Read the model definition and answer for the solid it produces. Units are mm, in the model's axes. A direction names the side the tool comes from. Coordinates: 2 decimals unless noted, no trailing zeros. Write each loop counter-clockwise with the first axis right and the second up, starting at its lowest first coordinate (ties: lowest second). Pieces come first, ordered by that corner, then holes.
(1) The part is cut by section C-C, the plane z = -15. Determine the outline of the cut face in (x, y), and give its area (3 significant figures).
(2) The part is cut by section B-B, the plane x = 15. Determine the outline of the cut face in (y, z), and give its area (3 significant figures).
(3) The part is cut by section D-D, the plane z = -6. Determine the outline of the cut face in (x, y).
(4) Given pin 1 (1.2 mm diameter, centred on y = 3, z = 9.5, fed in from +X); pin 2 (2 mm diameter, centred on y = 3.5, z = -4, fed in from -X); pin 3 (18.5 mm diameter, centred on x = -4, z = -3, fed in from +Y), each flat-ended and moving along its own axis, determine where each tip first touches the part or whether it passes through.
(5) The part is cut by section A-A, the plane y = 2.85. Determine the outline of the cut face in (x, z).
(6) Straight lines are drawn through the part: line 1 along X through (y, z) = (4.55, 15); line 2 along X through (y, z) = (0.75, 0); line 3 along X through (y, z) = (3.1, -15). For each, find the intervals that lie inside material, in ascending order.
(7) Which of the six approach directions +Z, -Z, +X, -X, +Y, -Y give full straight-line access (tool end or side, diameter ignored) to faces 4 (the flat face through (-20, 3, 0)), 5 (the cylindrical face through (-14.052, 3.472, 16.237)), 6 (the flat face through (0, 2, -19))?
(8) Determine the mould class of faces 1 (the flat face through (10, 4, -19)), 2 (the flat face through (26.9, 0.7, 10.8)), 3 (the cylindrical face through (14.052, 3.472, 13.763)) for opening direction Z: pulls with the +Z half, pulls with the -Z half, needs draft (parallel to the pull), parting line crosses it, or undercut.
```python
from build123d import *

# Parameters (mm, degrees)
SKETCH1_R           = 1.5
SKETCH1_R_2         = 2.5
BOSS_EXTRUDE1_DEPTH = 1.5
SKETCH2_W           = 40
SKETCH2_H           = 40
SKETCH2_R           = 1.5
SKETCH2_R_2         = 1.558204887
BOSS_EXTRUDE2_DEPTH = 4
SKETCH3_W           = 20
SKETCH3_H           = 3.5
CUT_EXTRUDE1_DEPTH  = 2
SKETCH4_W           = 20
SKETCH4_H           = 3.5
CUT_EXTRUDE2_DEPTH  = 2
FILLET1_R           = 3


with BuildPart() as part:
    # Sketch1 → Boss-Extrude1 (new body)
    with BuildSketch(Plane(origin=(0, 0, 0), x_dir=(1, 0, 0), z_dir=(0, 1, 0))):
        Polygon((-20, 20), (20, 20), (35, 0), (20, -20), (-20, -20), (-35, 0), align=None)
        with Locations(Location((-15, 15, 0), (0, 0, 270))):
            Circle(SKETCH1_R, mode=Mode.SUBTRACT)
        with Locations(Location((15, 15, 0), (0, 0, 270))):
            Circle(SKETCH1_R, mode=Mode.SUBTRACT)
        with Locations(Location((15, -15, 0), (0, 0, 90))):
            Circle(SKETCH1_R, mode=Mode.SUBTRACT)
        with Locations(Location((-15, -15, 0), (0, 0, 90))):
            Circle(SKETCH1_R, mode=Mode.SUBTRACT)
        with Locations(Location((-30, 0, 0), (0, 0, 270))):
            Circle(SKETCH1_R_2, mode=Mode.SUBTRACT)
        with Locations(Location((30, 0, 0), (0, 0, 90))):
            Circle(SKETCH1_R_2, mode=Mode.SUBTRACT)
    extrude(amount=BOSS_EXTRUDE1_DEPTH)

    # Sketch2 → Boss-Extrude2 (add)
    with BuildSketch(Plane(origin=(0, 1.5, 0), x_dir=(1, 0, 0), z_dir=(0, 1, 0))):
        Rectangle(SKETCH2_W, SKETCH2_H)
        with Locations(Location((-15, 15, 0), (0, 0, 270))):
            Circle(SKETCH2_R, mode=Mode.SUBTRACT)
        with Locations(Location((15, -15, 0), (0, 0, 270))):
            Circle(SKETCH2_R_2, mode=Mode.SUBTRACT)
        with Locations(Location((-15, -15, 0), (0, 0, 90))):
            Circle(SKETCH2_R_2, mode=Mode.SUBTRACT)
        with Locations(Location((15, 15, 0), (0, 0, 90))):
            Circle(SKETCH2_R, mode=Mode.SUBTRACT)
        with BuildLine():
            Line((-18.5, 11.429285786), (-18.5, -11.429285786))
            ThreePointArc((-18.5, -11.429285786), (-11.464466094, -11.464466094), (-11.429285786, -18.5))
            Line((-11.429285786, -18.5), (11.429285786, -18.5))
            ThreePointArc((11.429285786, -18.5), (11.464466094, -11.464466094), (18.5, -11.429285786))
            Line((18.5, -11.429285786), (18.5, 11.429285786))
            ThreePointArc((18.5, 11.429285786), (11.464466094, 11.464466094), (11.429285786, 18.5))
            Line((11.429285786, 18.5), (-11.429285786, 18.5))
            ThreePointArc((-11.429285786, 18.5), (-11.464466094, 11.464466094), (-18.5, 11.429285786))
        make_face(mode=Mode.SUBTRACT)
    extrude(amount=BOSS_EXTRUDE2_DEPTH)

    # Sketch3 → Cut-Extrude1 (cut)
    with BuildSketch(Plane.XY.offset(20)):
        with Locations((0, 3.75)):
            Rectangle(SKETCH3_W, SKETCH3_H)
    extrude(amount=-CUT_EXTRUDE1_DEPTH, mode=Mode.SUBTRACT)

    # Sketch4 → Cut-Extrude2 (cut)
    with BuildSketch(Plane(origin=(0, 0, -20), x_dir=(-1, 0, 0), z_dir=(0, 0, -1))):
        with Locations((0, 3.75)):
            Rectangle(SKETCH4_W, SKETCH4_H)
    extrude(amount=-CUT_EXTRUDE2_DEPTH, mode=Mode.SUBTRACT)

    # Fillet1
    fillet1_edges = [part.edges().sort_by_distance(p)[0] for p in [
        (-35, 0.75, 0),
        (35, 0.75, 0),
    ]]
    fillet(fillet1_edges, radius=FILLET1_R)


solid = part.part
```
Computed:
1. outline: (-23.75, 0) - (-16.5, 0) - (-16.5, 5.5) - (-20, 5.5) - (-20, 1.5) - (-23.75, 1.5) - close; (-13.5, 0) - (13.5, 0) - (13.5, 5.5) - (10, 5.5) - (10, 1.5) - (-10, 1.5) - (-10, 5.5) - (-13.5, 5.5) - close; (16.5, 0) - (23.75, 0) - (23.75, 1.5) - (20, 1.5) - (20, 5.5) - (16.5, 5.5) - close
1. area: 118 mm2
2. outline: (0, -20) - (5.5, -20) - (5.5, -16.5) - (0, -16.5) - close; (0, -13.5) - (5.5, -13.5) - (5.5, -10) - (1.5, -10) - (1.5, 10) - (5.5, 10) - (5.5, 13.44) - (1.5, 13.44) - (1.5, 13.5) - (0, 13.5) - close; (0, 16.5) - (1.5, 16.5) - (1.5, 16.56) - (5.5, 16.56) - (5.5, 20) - (0, 20) - close
2. area: 107 mm2
3. outline: (-30.5, 0) - (30.5, 0) - (30.5, 1.5) - (20, 1.5) - (20, 5.5) - (18.5, 5.5) - (18.5, 1.5) - (-18.5, 1.5) - (-18.5, 5.5) - (-20, 5.5) - (-20, 1.5) - (-30.5, 1.5) - close
4. pin 1: stops at x = 20
4. pin 2: stops at x = -20
4. pin 3: stops at y = 1.5
5. outline: (-20, -20) - (-10, -20) - (-10, -18.5) - (-11.43, -18.5) arc R5 ccw to (-18.5, -11.43) - (-18.5, 11.43) arc R5 ccw to (-11.43, 18.5) - (-10, 18.5) - (-10, 20) - (-20, 20) - close; (10, -20) - (20, -20) - (20, 20) - (10, 20) - (10, 18.5) - (11.43, 18.5) arc R5 ccw to (18.5, 11.43) - (18.5, -11.43) arc R5 ccw to (11.43, -18.5) - (10, -18.5) - close; hole circle Ø3.12 at (-15, 15); hole circle Ø3 at (-15, -15); hole circle Ø3.12 at (15, 15); hole circle Ø3 at (15, -15)
6. line 1: x = -20 to -16.56, -13.44 to -10, 10 to 13.44, 16.56 to 20
6. line 2: x = -34.25 to -32.5, -27.5 to 27.5, 32.5 to 34.25
6. line 3: x = -20 to -16.5, -13.5 to -10, 10 to 13.5, 16.5 to 20
7. face 4: +Z, -Z, -X, +Y
7. face 5: +Y
7. face 6: +Z, -Z, +Y
8. face 1: needs draft
8. face 2: pulls with the +Z half
8. face 3: undercut
